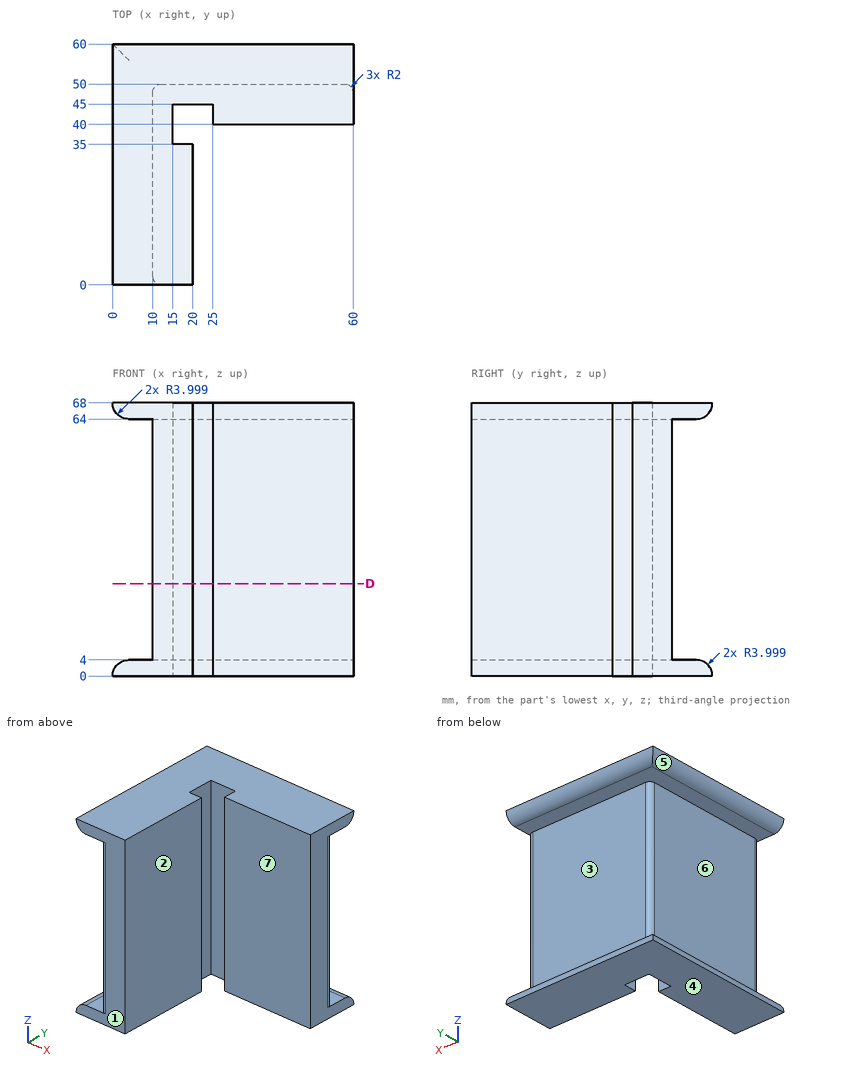
Input: dimensioned drawing with shaded views. Units: mm. Origin: part minimum x, y, z. A direction names the side the tool comes from. Coordinates: 2 decimals unless noted, no trailing zeros. Loops run counter-clockwise (first coordinate to the right, second up) from the corner with the lowest first, then second, coordinate; pieces in that order, holes last. Notation, with made-up numbers: (9, 55) -> (41, 55) arc R35 ccw to (41, 93) -> close; hole circle Ø8 at (45, -38). An arc over 180 degrees is marked (long way). Use a Markdown table: item, result. Add a question column.
(1) Access query for the marked faces 1, 2 and 3. Directions: +Z, -Z, +X, -X, +Y, -Y. A direction counts if a zero-diameter tool reaches every point of the face in a straight line with its end or side. Return the directions, or none.
(2) Section query D-D, the plane z = 23. Return loops of the section in (x, y).
(3) Mould query, pull axis Z, two halves, no side actions, for the marked faces 4, 5, 6 and 7. Classes: pulls with the +Z half, pulls with the -Z half, needs draft (parallel to the pull), parting line crosses it, or undercut.
(4) Pin query (flat end, axial travel): pin 1 Ø8 at (y, z) = (45, 29) entering from -X; pin 2 Ø8 at (y, z) = (37, 59.5) entering from +X; pin 3 Ø17.5 at (y, z) = (14, 22) entering from +X; pin 4 Ø3 at (x, z) = (33, 16) entering from -Y. Return the tip coordinate at first contact, or that it passes through.
(5) Line query: line 1 along Y through (x, z) = (18, 20.5); line 2 along Z through (x, y) = (8.5, 6); line 3 along Y through (x, z) = (56.5, 15). Output: solid intervals per line, ascending.
Answer:
| question | item | result |
|---|---|---|
| 1 | face 1 | +Z, -Z, +X, -X, -Y |
| 1 | face 2 | +Z, -Z, +X, -Y |
| 1 | face 3 | +X, -X, +Y |
| 2 | outline | (10, 2) arc R2 ccw to (12, 0) -> (20, 0) -> (20, 35) -> (15, 35) -> (15, 45) -> (25, 45) -> (25, 40) -> (60, 40) -> (60, 48) arc R2 ccw to (58, 50) -> (12, 50) arc R2 ccw to (10, 48) -> close |
| 3 | face 4 | pulls with the -Z half |
| 3 | face 5 | undercut |
| 3 | face 6 | undercut |
| 3 | face 7 | needs draft |
| 4 | pin 1 | stops at x = 10 |
| 4 | pin 2 | stops at x = 60 |
| 4 | pin 3 | stops at x = 20 |
| 4 | pin 4 | stops at y = 40 |
| 5 | line 1 | y = 0 to 35, 45 to 50 |
| 5 | line 2 | z = 0 to 4, 64 to 68 |
| 5 | line 3 | y = 40 to 50 |
